from build123d import *

# Parameters (mm, degrees)
CROQUIS1_W              = 1
CROQUIS1_H              = 2
SALIENTE_EXTRUIR1_START = -1
SALIENTE_EXTRUIR1_DEPTH = 1
MATRIZC1_COUNT          = 4


with BuildPart() as part:
    # Croquis1 → Revolución1 (revolve)
    with BuildSketch(Plane.XY, mode=Mode.PRIVATE) as revoluci_n1_sk:
        with Locations((11.05, 0)):
            Rectangle(CROQUIS1_W, CROQUIS1_H)
    revolve(revoluci_n1_sk.sketch.rotate(Axis((0, 18.472461404, 0), (0, -1, 0)), 90), axis=Axis((0, 18.472461404, 0), (0, -1, 0)))

    # Croquis2 → Saliente-Extruir1 (add)
    with BuildSketch(Plane(origin=(0, 0, 0), x_dir=(1, 0, 0), z_dir=(0, 1, 0)).offset(SALIENTE_EXTRUIR1_START)):
        Polygon((-5, -10.411652126), (-5, -14.6), (5, -14.6), (5, -10.411652126), (3.8, -10.411652126), (3.8, -10.90699317), (3.8, -13.6), (-3.8, -13.6), (-3.8, -10.90699317), (-3.8, -10.411652126), align=None)
    saliente_extruir1 = extrude(amount=SALIENTE_EXTRUIR1_DEPTH)

    # MatrizC1: Saliente-Extruir1 ×4 about axis
    matrizc1_axis = Axis((0, 0, 0), (0, 1, 0))
    for i in range(1, MATRIZC1_COUNT):
        add(saliente_extruir1.rotate(matrizc1_axis, i * 360 / MATRIZC1_COUNT))


solid = part.part
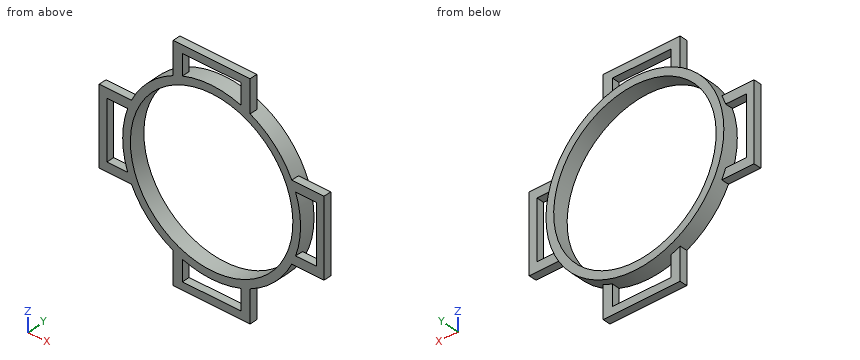
Here's how the part is built. I have some questions about the finished solid (model axes, mm). Coordinates: 2 decimals unless noted, no trailing zeros. Order: outer loops, then holes, each group sorted by start corner. A loop starts at its lowest first (then second) coordinate and runs counter-clockwise, first axis right, second up. Notation, with made-up numbers: (31, -3.5) -> (75, -3.5) arc R27 cw to (75, 27.5) -> close; hole circle Ø2 at (36, 38.5). An arc over 180 degrees is marked (long way). Answer in a Markdown table with one row per item.
(1) I want a section at D-D on z = 12.5. List the corners of the cut face in (x, y) for me.
Answer key:
| item | result |
|---|---|
| outline | (-5, -1) -> (-3.8, -1) -> (-3.8, 0) -> (-5, 0) -> close; (3.8, -1) -> (5, -1) -> (5, 0) -> (3.8, 0) -> close |
(2) I want a section at C-C on y = -0.55. Count the separate pieces of the cut face and the enclosed holes in it, then the cut area to 3 significant figures.
Answer key:
| item | result |
|---|---|
| separate pieces | 1 |
| enclosed holes | 5 |
| area | 138 mm^2 |
(3) I want a section at A-A on z = 0. List the corners of the cut face in (x, y) for me.
Answer key:
| item | result |
|---|---|
| outline | (-14.6, -1) -> (-13.6, -1) -> (-13.6, 0) -> (-14.6, 0) -> close; (-11.55, -1) -> (-10.55, -1) -> (-10.55, 1) -> (-11.55, 1) -> close; (10.55, -1) -> (11.55, -1) -> (11.55, 1) -> (10.55, 1) -> close; (13.6, -1) -> (14.6, -1) -> (14.6, 0) -> (13.6, 0) -> close |
(4) Please list where these lines run through material, in increasing order: probe 1 along X at (y, z) = (-0.25, 0); probe 2 along X at (y, z) = (-0.2, 13.25).
Answer key:
| item | result |
|---|---|
| probe 1 | -14.6 to -13.6, -11.55 to -10.55, 10.55 to 11.55, 13.6 to 14.6 |
| probe 2 | -5 to -3.8, 3.8 to 5 |
(5) I want a section at B-B on x = 0. List the corners of the cut face in (y, z) for me.
Answer key:
| item | result |
|---|---|
| outline | (-1, -14.6) -> (0, -14.6) -> (0, -13.6) -> (-1, -13.6) -> close; (-1, -11.55) -> (1, -11.55) -> (1, -10.55) -> (-1, -10.55) -> close; (-1, 10.55) -> (1, 10.55) -> (1, 11.55) -> (-1, 11.55) -> close; (-1, 13.6) -> (0, 13.6) -> (0, 14.6) -> (-1, 14.6) -> close |
(6) Will these pins go through, and if not, where does the flat tip stop? pin 1 Ø1.1 at (x, y) = (13.5, -0.5) entering from -Z; pin 2 Ø0.8 at (y, z) = (-0.5, 12.5) entering from -X; pin 3 Ø0.8 at (y, z) = (-0.5, -13) entering from +X; pin 4 Ø6 at (x, z) = (-7.5, 3.5) entering from +Y.
Answer key:
| item | result |
|---|---|
| pin 1 | z = -5 |
| pin 2 | x = -5 |
| pin 3 | x = 5 |
| pin 4 | y = 1 |
